Geometry: see drawing. Coordinates: mm, zero at the bounding-box minimum. A direction names the side the tool comes from. Round coordinates to 2 decimals unless told otherwise and drop trailing zeros. Loops run counter-clockwise (first coordinate to the right, second up) from the corner with the lowest first, then second, coordinate; pieces in that order, holes last. Notation, with made-up numbers: (48.25, 75) - (85.25, 75) arc R17 cw to (85.25, 82) - close; hole circle Ø5 at (87.25, 47). An arc over 180 degrees is marked (long way). Write item = value, one per line. Start each with the question number.
Item 1: Section C-C (y = 19.5). Return loops of the section in (x, z).
Item 2: Line query: line 1 (Y direction, x = 3.5, z = 2.05); line 2 (X direction, y = 5, z = 0.85); line 3 (Y direction, x = 32.5, z = 1.05). Output: solid intervals per line, ascending. Write a range as from..to.
Item 3: Draft query along X for the marked faces 1, 2 and 3. Return one class per face: pulls with the +X half, pulls with the -X half, needs draft (parallel to the pull), parting line crosses it, or undercut.
Item 4: First-contact query: pin 1 (1.6 mm diameter, centred on x = 1, y = 9, fed in from -Z); pin 2 (3.5 mm diameter, centred on x = 3.5, y = 19.5, fed in from +Z); pin 3 (0.8 mm diameter, centred on x = 16.5, z = 3.5, fed in from +Y) (3 decimals). Flat tips, straight axial feed; report the tip coordinate or a pass-through.
Item 5: Access query for the marked faces 4, 5 and 6. Directions: +Z, -Z, +X, -X, +Y, -Y. A direction counts if a zero-diameter tool reaches every point of the face in a straight line with its end or side. Return the directions, or none.
Item 6: Section A-A (y = 10). Return loops of the section in (x, z), plus the area to 3 significant figures.
Item 7: Section D-D (z = 2.45). Return loops of the section in (x, y), plus the area to 3 significant figures.
Item 8: Section B-B (x = 3.5). Return loops of the section in (y, z).
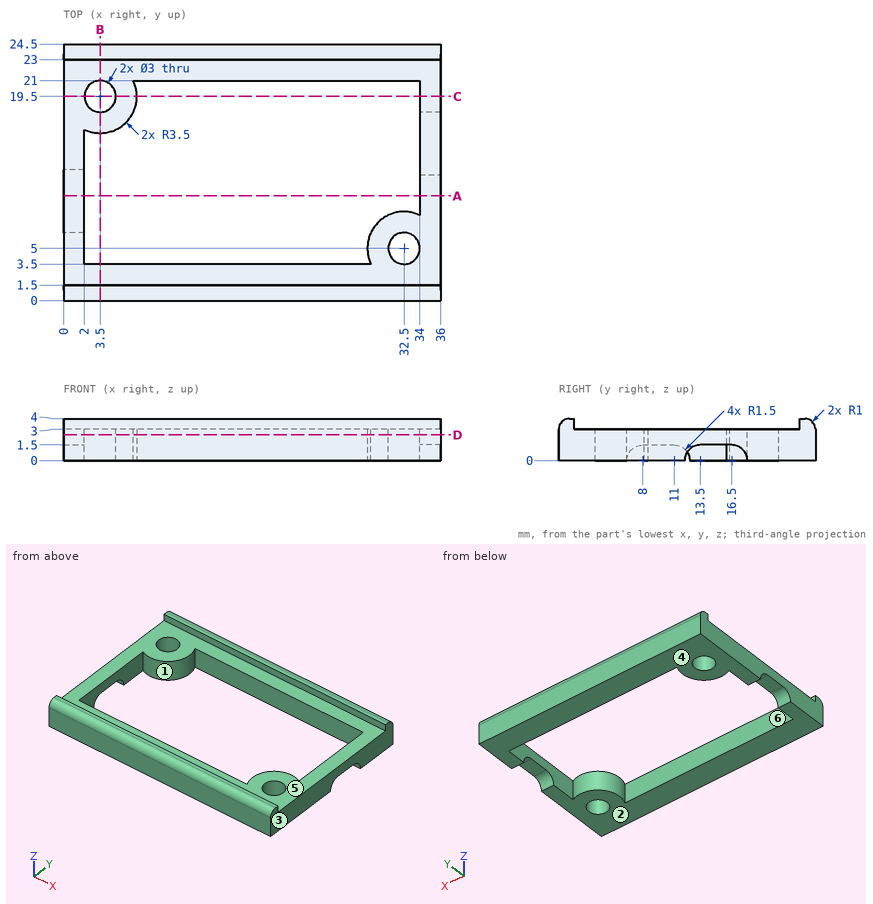
Taken from the geometry:
q1.outline = (0, 0) - (2, 0) - (2, 3) - (0, 3) - close; (5, 0) - (7, 0) - (7, 3) - (5, 3) - close; (34, 0) - (36, 0) - (36, 3) - (34, 3) - close
q2.line_1 = 0..3.5, 16..18, 21..24.5
q2.line_2 = 0..2, 29..31, 34..36
q2.line_3 = 0..3.5, 6.5..8.5, 21..24.5
q3.face_1 = undercut
q3.face_2 = needs draft
q3.face_3 = pulls with the +X half
q4.pin_1 = 1.5
q4.pin_2 = 3
q4.pin_3 = 24.495
q5.face_4 = -Z, +X, -X, +Y, -Y
q5.face_5 = +Z, +X, -X
q5.face_6 = +Z, -Z
q6.outline = (0, 1.5) - (2, 1.5) - (2, 3) - (0, 3) - close; (34, 0) - (36, 0) - (36, 3) - (34, 3) - close
q6.area = 9.00 mm^2
q7.outline = (0, 0) - (36, 0) - (36, 24.5) - (0, 24.5) - close; hole (2, 3.5) - (29.34, 3.5) arc R3.5 cw to (34, 8.16) - (34, 21) - (6.66, 21) arc R3.5 cw to (2, 16.34) - close; hole circle Ø3 at (3.5, 19.5); hole circle Ø3 at (32.5, 5)
q7.area = 352 mm^2
q8.outline = (0, 0) - (3.5, 0) - (3.5, 3) - (1.5, 3) - (1.5, 4) - (1, 4) arc R1 ccw to (0, 3) - close; (16, 0) - (18, 0) - (18, 3) - (16, 3) - close; (21, 0) - (24.5, 0) - (24.5, 3) arc R1 ccw to (23.5, 4) - (23, 4) - (23, 3) - (21, 3) - close
